Part print with two shaded views. Sizes in mm from the minimum x, y, z corner. Round coordinates to 2 decimals unless told otherwise and drop trailing zeros. Loops run counter-clockwise (first coordinate to the right, second up) from the corner with the lowest first, then second, coordinate; pieces in that order, holes last.
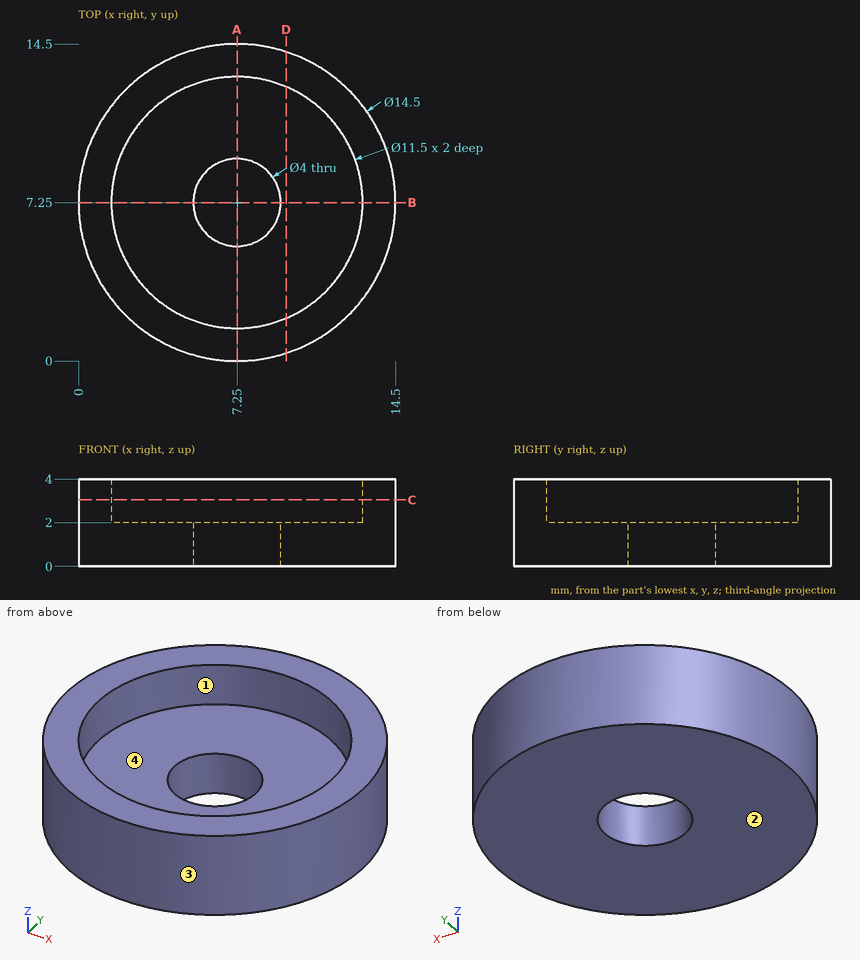
Item 1: Cut at C-C (z = 3.05). List the corners of the cut face in (x, y), plus the area to 3 significant figures.
Verdict:
outline: circle Ø14.5 at (7.25, 7.25); hole circle Ø11.5 at (7.25, 7.25)
area: 61.3 mm2
Item 2: Cut at D-D (x = 9.5). List the corners of the cut face in (y, z).
Verdict:
outline: (0.36, 0) - (14.14, 0) - (14.14, 4) - (12.54, 4) - (12.54, 2) - (1.96, 2) - (1.96, 4) - (0.36, 4) - close
Item 3: Mould opens along X. For the marked faces 1, 2, 3 and 4 say: released by +X, released by -X, zero draft, split by the parting line, or undercut.
Verdict:
face 1: undercut
face 2: zero draft
face 3: split by the parting line
face 4: undercut
Item 4: Flat gauge pin, fed straight in: P1, Ø6.5, axis at x = 7.25, y = 7.25, coming from the +Z side. Where does the tip first touch, or does it go through?
Verdict:
P1: stops at z = 2
Item 5: Cut at A-A (x = 7.25). List the corners of the cut face in (y, z).
Verdict:
outline: (0, 0) - (5.25, 0) - (5.25, 2) - (1.5, 2) - (1.5, 4) - (0, 4) - close; (9.25, 0) - (14.5, 0) - (14.5, 4) - (13, 4) - (13, 2) - (9.25, 2) - close
Item 6: Wall check: L1, parallel to Y at x = 7.25, z = 2.7; L2, parallel to Y at x = 7.25, z = 1.05; L3, parallel to X at y = 7, z = 3.5. Give the ranges that are in metal, low to high.
Verdict:
L1: y = 0 to 1.5, 13 to 14.5
L2: y = 0 to 5.25, 9.25 to 14.5
L3: x = 0 to 1.51, 12.99 to 14.5
